Geometry: final body of the model. Coordinates: model frame, mm. Round coordinates to 2 decimals unless told otherwise and drop trailing zeros. Loops run counter-clockwise (first coordinate to the right, second up) from the corner with the lowest first, then second, coordinate; pieces in that order, holes last. Notation, with made-up numbers: M 77.25,21 L 116.25,21 A15 cw 116.25,42 Z; hole C -7.5,25.5 d4. An arc over 180 degrees is marked long. Answer as a JSON object with one key per item and string values.
from build123d import *

# Parameters (mm, degrees)
F1_DEPTH = 38.1
F2_DEPTH = 38.1
F3_DEPTH = 38.1


with BuildPart() as f1:
    # F0 (on Front) → F1 (new body)
    with BuildSketch(Plane.XZ):
        Polygon((159.819499, 0), (248.719499, 0), (248.719499, 88.9), align=None)
        Polygon((-158.442501, 0), (159.819499, 0), (248.719499, 88.9), (-247.342501, 88.9), align=None)
        Polygon((-247.342501, 0), (-158.442501, 0), (-247.342501, 88.9), align=None)
    extrude(amount=F1_DEPTH)

    # F0 (on Front) → F2 (cut)
    with BuildSketch(Plane.XZ):
        Polygon((-247.342501, 0), (-158.442501, 0), (-247.342501, 88.9), align=None)
    extrude(amount=F2_DEPTH, mode=Mode.SUBTRACT)

    # F0 (on Front) → F3 (cut)
    with BuildSketch(Plane.XZ):
        Polygon((159.819499, 0), (248.719499, 0), (248.719499, 88.9), align=None)
    extrude(amount=F3_DEPTH, mode=Mode.SUBTRACT)


solid = f1.part
1) Section query A-A (y = -7.5). Return the cut outline in (x, z), and give its area (3 significant figures).
Results:
{"outline": "M -247.34,88.9 L -158.44,0 L 159.82,0 L 248.72,88.9 Z", "area": "36,200 mm2"}
2) Pin query (flat end, axial travel): P1, Ø4, axis at y = -23, z = 63, coming from the +X side. Return the tip coordinate at first contact, or that it passes through.
Results:
{"P1": "x = 224.82"}
3) Ray query, line 1 (Z direction, x = -220, y = -22.5); line 2 (X direction, y = -7.5, z = 14); line 3 (X direction, y = -35, z = 47.5). Return the intervals inside material, ascending.
Results:
{"line 1": "61.56 to 88.9", "line 2": "-172.44 to 173.82", "line 3": "-205.94 to 207.32"}
4) Section query B-B (z = 19). Return the cut outline in (x, y), and give its area (3 significant figures).
Results:
{"outline": "M -177.44,-38.1 L 178.82,-38.1 L 178.82,0 L -177.44,0 Z", "area": "13,600 mm2"}
